Autodesk Inventor part; units mm, degrees
ref_plane "YZ Plane" through (0, 0, 0) normal (1, 0, 0) x (0, 1, 0)
ref_plane "XZ Plane" through (0, 0, 0) normal (0, 1, 0) x (-1, 0, 0)
ref_plane "XY Plane" through (0, 0, 0) normal (0, 0, 1) x (1, 0, 0)
sketch "Sketch1" plane through (0, 0, 0) normal (0, 0, 1) x (1, 0, 0)
  line L0 (0, 0) -> (19.05, 0)
  line L1 (19.05, 0) -> (19.05, -31.75)
  line L2 (19.05, -31.75) -> (0, -31.75)
  line L3 (0, -31.75) -> (0, 0)
  circle A0 centre (9.525, -15.875) radius 3.175
  line L4 (19.05, -31.75) -> (44.45, -31.75)
  line L5 (44.45, -31.75) -> (44.45, 0)
  line L6 (44.45, 0) -> (19.05, 0)
  line L7 (19.05, 0) -> (19.05, -31.75)
  circle A1 centre (31.75, -15.875) radius 3.175
  dimension "d0" = 19.05
  dimension "d1" = 31.75
  dimension "d2" = 6.35
  dimension "d5" = 25.4
extrude "Extrusion1" add sketch "Sketch1" along normal blind 2.54 contours L0 L1 L2 L3
extrude "Extrusion2" cut sketch "Sketch1" along normal blind 2.54 contours L6 L5 L4 L1
extrude "Extrusion3" add sketch "Sketch1" along normal blind 2.54 contours L6 L5 L4 L1
fillet "Fillet1" radius 3.175 1 edges at (0, 0, 1.27)
fillet "Fillet2" radius 3.175 1 edges at (0, -31.75, 1.27)
sketch "Sketch3" plane through (0, 0, 2.54) normal (0, 0, 1) x (1, 0, 0)
  circle A0 centre (31.75, -15.875) radius 3.175
  circle A1 centre (31.75, -41.275) radius 3.178
  line L0 (44.45, -31.75) -> (19.05, -31.75)
  line L1 (19.05, -31.75) -> (19.05, -50.8)
  line L2 (19.05, -50.8) -> (44.45, -50.8)
  line L3 (44.45, -50.8) -> (44.45, -31.75)
  point P0 (0, 0)
  dimension "d12" = 25.4
  dimension "d13" = 19.05
extrude "Extrusion4" add sketch "Sketch3" against normal blind 2.54 contours L3 L2 L1 L0
properties part number "Pneumatic Spring attach Point"
Could you check a few things on this model? Use its own coordinates, in mm. A direction names the side the tool comes from. Give positions to 0.01 mm unless a question says otherwise; leave off trailing zeros. Loops run counter-clockwise (first coordinate to the right, second up) from the corner with the lowest first, then second, coordinate; pieces in that order, holes last. Notation, with made-up numbers: (-25.5, 35.25) -> (11.5, 35.25) arc R26 ccw to (11.5, 69.25) -> close; hole circle Ø3 at (-35.75, 22). An arc over 180 degrees is marked (long way). Put each result on its own line as item: value.
(1) Please list where these lines run through material, in increasing order: probe 1 along Y at (x, z) = (31.75, 1.15); probe 2 along Y at (x, z) = (33.5, 1.85); probe 3 along Y at (x, z) = (16, 1.9). Write a range as [from, to].
Computed:
probe 1: [-50.8, -44.45], [-38.1, -19.05], [-12.7, 0]
probe 2: [-50.8, -43.93], [-38.62, -18.52], [-13.23, 0]
probe 3: [-31.75, 0]
(2) Imagine slicing it at B-B on x = 31.75. Write out the boundary of the cut face in (y, z), plus the area to 3 significant figures.
Computed:
outline: (-50.8, 0) -> (-44.45, 0) -> (-44.45, 2.54) -> (-50.8, 2.54) -> close; (-38.1, 0) -> (-19.05, 0) -> (-19.05, 2.54) -> (-38.1, 2.54) -> close; (-12.7, 0) -> (0, 0) -> (0, 2.54) -> (-12.7, 2.54) -> close
area: 96.8 mm^2
(3) I'm going to push flat-ended pins straight in: pin 1 Ø1.3 at (y, z) = (-39, 1.5) entering from -X; pin 2 Ø1 at (x, z) = (14, 2) entering from -Y. Where does each tip first touch, or does it pass through?
Computed:
pin 1: x = 19.05
pin 2: y = -31.75
(4) Imagine slicing it at C-C on z = 1.65. Write out the boundary of the cut face in (x, y) (3 decimals), plus the area to 3 significant figures.
Computed:
outline: (0, -28.575) arc R3.175 ccw to (3.175, -31.75) -> (19.05, -31.75) -> (19.05, -50.8) -> (44.45, -50.8) -> (44.45, 0) -> (3.175, 0) arc R3.175 ccw to (0, -3.175) -> close; hole circle Ø6.35 at (9.525, -15.875); hole circle Ø6.356 at (31.75, -41.275); hole circle Ø6.35 at (31.75, -15.875)
area: 1,800 mm^2
(5) For faces 1 (the face through (19.05, -41, 1)), 2 (the face through (22, -19, 0)), which set-ups out of +Z, -Z, +X, -X, +Y, -Y let a thin tool reach every point of the face, with its end or its side?
Computed:
face 1: +Z, -Z, -X, -Y
face 2: -Z, +X, -X, +Y, -Y
(6) Thinking about a two-plate mould opening in Y: for faces 3 (the face through (44.45, -26, 1)), 4 (the face through (34.78, -40.32, 1.29)), 5 (the face through (0.91, -30.8, 1.29)), which applies, pulls with the +Y half, pulls with the -Y half, needs draft (parallel to the pull), parting line crosses it, or undercut?
Computed:
face 3: needs draft
face 4: undercut
face 5: pulls with the -Y half
(7) Imagine slicing it at A-A on x = 8.5. Write out the boundary of the cut face in (y, z), plus the area to 3 significant figures.
Computed:
outline: (-31.75, 0) -> (-18.88, 0) -> (-18.88, 2.54) -> (-31.75, 2.54) -> close; (-12.87, 0) -> (0, 0) -> (0, 2.54) -> (-12.87, 2.54) -> close
area: 65.4 mm^2
